The figure shows three views and two pictorial views of one solid part (mm, origin at its lowest corner). Answer the questions. Coordinates: 2 decimals unless noted, no trailing zeros. Write each loop counter-clockwise with the first axis right and the second up, starting at its lowest first coordinate (ties: lowest second). Pieces come first, ordered by that corner, then holes. Notation, with made-up numbers: (17, 64) - (62, 64) arc R28 ccw to (62, 96) - close; hole circle Ø5 at (52.25, 74). An arc over 180 degrees is marked (long way). Use a Markdown table: item, result. Add a question column.
(1) The part is cut by section A-A, the plane y = 2. Give the vertices of the cut face in (x, z) (1 decimal).
(2) Given pin 1 Ø5 at (y, z) = (6.5, 30) entering from -X; pin 2 Ø2 at (x, y) = (25.5, 6.5) entering from +Z; pin 3 Ø2 at (y, z) = (2, 20.5) entering from +X, each flat-ended and moving along its own axis, determine where each tip first touches the part or whether it passes through.
(3) Find the intervals of material crossed by line 1 (X direction, y = 8.25, z = 13.5); line 2 (Z direction, x = 11, y = 6.5); line 3 (Z direction, x = 4.5, y = 2), in increasing order. Write a range as from..to.
(4) The part is cut by section C-C, the plane z = 11.5. Give the vertices of the cut face in (x, y) (1 decimal), then the cut area to 3 significant figures.
(5) The part is cut by section B-B, the plane x = 27. Give the vertices of the cut face in (y, z), then the cut area to 3 significant figures.
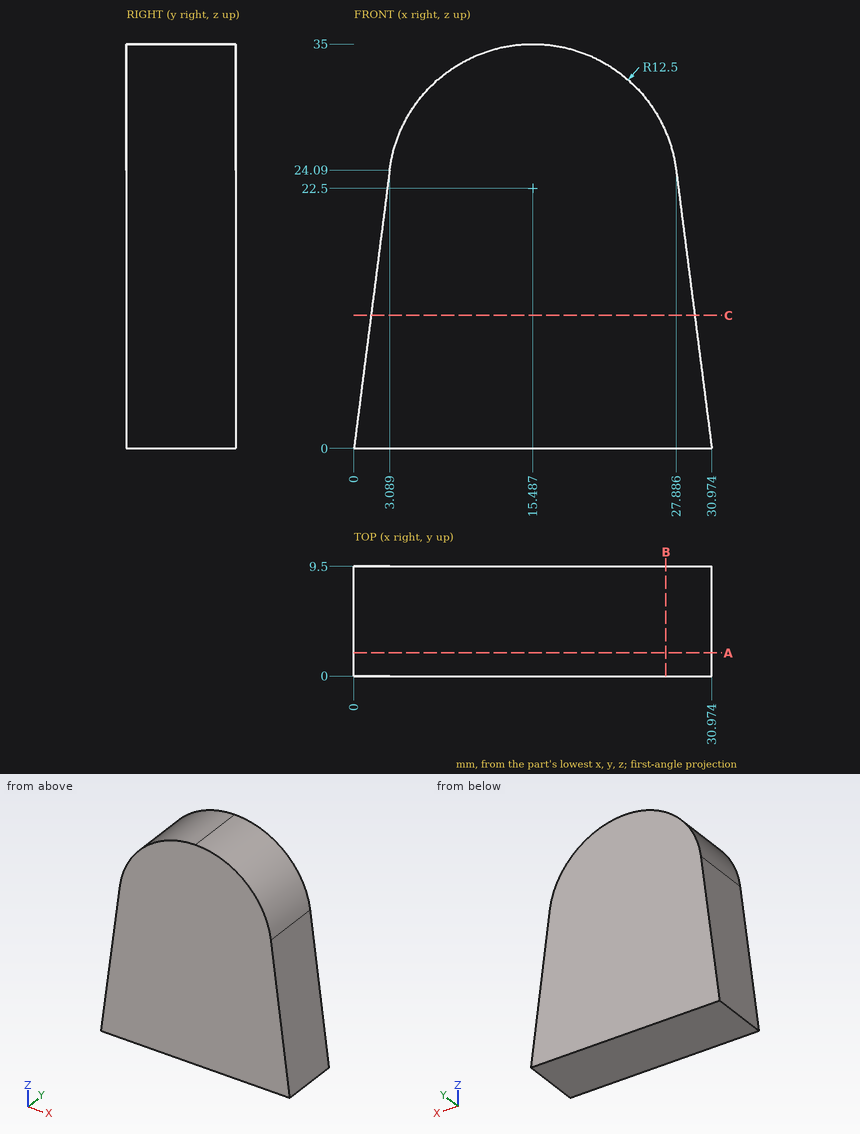
Model answer:
| question | item | result |
|---|---|---|
| 1 | outline | (0, 0) - (31, 0) - (27.9, 24.1) arc R12.5 ccw to (15.5, 35) arc R12.5 ccw to (3.1, 24.1) - close |
| 2 | pin 1 | x = 4.03 |
| 2 | pin 2 | z = 31.16 |
| 2 | pin 3 | x = 28.47 |
| 3 | line 1 | 1.73..29.24 |
| 3 | line 2 | 0..34.17 |
| 3 | line 3 | 0..28.46 |
| 4 | outline | (1.5, 0) - (29.5, 0) - (29.5, 9.5) - (1.5, 9.5) - close |
| 4 | area | 266 mm^2 |
| 5 | outline | (0, 0) - (9.5, 0) - (9.5, 27.37) - (0, 27.37) - close |
| 5 | area | 260 mm^2 |
